Work out the finished part from the listing and answer in its coordinate system (mm). A direction names the side the tool comes from. Round coordinates to 2 decimals unless told otherwise and drop trailing zeros. Order: outer loops, then holes, each group sorted by start corner. A loop starts at its lowest first (then second) coordinate and runs counter-clockwise, first axis right, second up.
Autodesk Inventor part; units mm, degrees
ref_plane "YZ Plane" through (0, 0, 0) normal (1, 0, 0) x (0, 1, 0)
ref_plane "XZ Plane" through (0, 0, 0) normal (0, 1, 0) x (-1, 0, 0)
ref_plane "XY Plane" through (0, 0, 0) normal (0, 0, 1) x (1, 0, 0)
sketch "Sketch1" plane through (0, 0, 0) normal (0, 0, 1) x (1, 0, 0)
  line L0 (0, 0) -> (0, 365)
  line L1 (0, 365) -> (597.3065, 0)
  line L2 (597.3065, 0) -> (0, 0)
  dimension "d0" = 365
  dimension "d1" = 700
extrude "Extrusion1" add sketch "Sketch1" along normal blind 20
sketch "Sketch2" plane through (0, 0, 20) normal (0, 0, 1) x (1, 0, 0)
  line L0 (30.8422, 26.0696) -> (30.8422, 311.5961)
  line L1 (0, 365) -> (0, 0)
  line L2 (30.8422, 311.5961) -> (501.2951, 26.0696)
  line L3 (501.2951, 26.0696) -> (30.8422, 26.0696)
extrude "Extrusion2" cut sketch "Sketch2" against normal blind 161.75
sketch "Sketch3" plane through (0, 0, 20) normal (0, 0, 1) x (1, 0, 0)
  line L0 (0, 365) -> (597.3065, 0)
  line L1 (0, 365) -> (0, 393.2795)
  line L2 (0, 393.2795) -> (643.5846, 0)
  line L3 (597.3065, 0) -> (643.5846, 0)
  point P0 (0, 0)
extrude "Extrusion3" add sketch "Sketch3" against normal blind 4
sketch "Sketch4" plane through (0, 0, 0) normal (0, 0, -1) x (-1, 0, 0)
  line L0 (-597.3065, 0) -> (0, 0)
  line L1 (-643.5846, 0) -> (-597.3065, 0)
  line L2 (-597.3065, 0) -> (-643.5846, 0)
  line L3 (0, 365) -> (0, 393.2795)
  line L4 (-643.5846, 0) -> (0, 393.2795)
  line L5 (0, 393.2795) -> (0, 365)
  line L6 (0, 365) -> (-597.3065, 0)
extrude "Extrusion4" add sketch "Sketch4" against normal blind 4
sketch "Sketch5" plane through (0, 0, 0) normal (0, -1, 0) x (1, 0, 0)
  line L0 (597.3065, 4) -> (643.5846, 4)
  line L1 (643.5846, 20) -> (643.5846, 16)
  line L2 (643.5846, 4) -> (643.5846, 16)
  line L3 (597.3065, 4) -> (597.3065, 16)
  line L4 (643.5846, 16) -> (597.3065, 16)
  line L5 (597.3065, 16) -> (597.3065, 4)
  point P0 (0, 0)
extrude "Extrusion5" add sketch "Sketch5" against normal blind 2.75
sketch "Sketch6" plane through (643.5846, 0, 16) normal (1, 0, 0) x (0, 0, -1)
  line L0 (-4, 0) -> (-4, 393.2795)
  line L1 (16, 0) -> (-4, 0)
  line L2 (-4, 0) -> (-4, 15)
  line L3 (-4, 15) -> (16, 15)
  line L4 (16, 15) -> (16, 0)
  dimension "d12" = 15
extrude "Extrusion6" add sketch "Sketch6" against normal blind 5
sketch "Sketch7" plane through (0, 0, 0) normal (-1, 0, 0) x (0, 0, 1)
  line L0 (0, 0) -> (0, 393.2795)
  line L1 (20, 3.0554) -> (20, 393.2795)
  line L2 (0, 393.2795) -> (20, 393.2795)
  line L3 (20, 393.2795) -> (20, 363.4031)
  line L4 (20, 363.4031) -> (0, 363.4031)
  line L5 (0, 363.4031) -> (0, 393.2795)
extrude "Extrusion7" add sketch "Sketch7" against normal blind 5
Item 1: Find section C-C (y = 305). Write down the section's boundary in (x, z).
Item 2: A tool of negligible diameter and unlimited length cuts with its end or side. For faces 1 (the face through (30.842, 167, 10)), 2 (the face through (618, 2.75, 10)), 3 (the face through (643.585, 8, 10)), from which of +Z, -Z, +X, -X, +Y, -Y can it reach the whole face along a straight path? Write none if from no direction.
Item 3: Find section D-D (x = 522). Write down the section's boundary in (y, z), plus the area to 3 significant figures.
Item 4: Find the intervals of material crossed by line 1 along X through (y, z) = (194, 13.5); line 2 along X through (y, z) = (241.5, 18); line 3 along Y through (x, z) = (385, 18.5) (3 decimals), in increasing order.
Item 5: Find section B-B (x = 287.5). Write down the section's boundary in (y, z).
Item 6: For a pull along Y with two mould halves and no side action, classify faces 4 (the face through (262.78, 170.83, 10.14)), 5 (the face through (326.23, 193.93, 1.97)), 6 (the face through (5, 379, 10)) as released by +Y, released by -Y, zero draft, split by the parting line, or undercut.
Item 7: Given pin 1 (6 mm diameter, centred on y = 378.5, z = 5.5, fed in from +X); pin 2 (12 mm diameter, centred on x = 226, z = 8, fed in from -Y); pin 3 (1.5 mm diameter, centred on y = 303.5, z = 10.5, fed in from +X); pin 4 (6 mm diameter, centred on x = 257.5, z = 8, fed in from +Y), each flat-ended and moving along its own axis, determine where each tip first touches the part or whether it passes through.
Model answer:
1. outline: (0, 0) - (30.84, 0) - (30.84, 20) - (0, 20) - close; (41.71, 0) - (144.47, 0) - (144.47, 4) - (98.19, 4) - (98.19, 16) - (144.47, 16) - (144.47, 20) - (41.71, 20) - close
2. face 1: +Z, -Z
2. face 2: +Y
2. face 3: +Z, -Z, +X, +Y, -Y
3. outline: (0, 0) - (74.3, 0) - (74.3, 4) - (46.02, 4) - (46.02, 16) - (74.3, 16) - (74.3, 20) - (0, 20) - close
3. area: 1,150 mm2
4. line 1: x = 0 to 30.84, 224.6 to 279.83
4. line 2: x = 0 to 30.84, 146.34 to 248.38
4. line 3: y = 0 to 26.07, 96.651 to 158.015
5. outline: (0, 0) - (26.07, 0) - (26.07, 20) - (0, 20) - close; (155.83, 0) - (217.59, 0) - (217.59, 4) - (189.32, 4) - (189.32, 16) - (217.59, 16) - (217.59, 20) - (155.83, 20) - close
6. face 4: undercut
6. face 5: released by +Y
6. face 6: zero draft
7. pin 1: stops at x = 28.44
7. pin 2: stops at y = 0
7. pin 3: stops at x = 101.87
7. pin 4: stops at y = 209.48
